Autodesk Fusion 360 part; units mm, degrees
sketch "Sketch1" plane through (0, 0, 0) normal (0, 0, 1) x (1, 0, 0)
  line L0 (4, -7) -> (-4, -7)
  line L1 (-4, -7) -> (-4, 7)
  line L2 (-4, 7) -> (4, 7)
  line L3 (4, 7) -> (4, -7)
  line L4 (4, -7) -> (-4, 7) construction
  line L5 (-4, -7) -> (4, 7) construction
  line L6 (0.5, -0.1) -> (-0.5, -0.1)
  line L7 (-0.5, -0.1) -> (-0.5, 0.1)
  line L8 (-0.5, 0.1) -> (0.5, 0.1)
  line L9 (0.5, 0.1) -> (0.5, -0.1)
  line L10 (0.5, -0.1) -> (-0.5, 0.1) construction
  line L11 (-0.5, -0.1) -> (0.5, 0.1) construction
  line L12 (0.5, -6.6) -> (-0.5, -6.6)
  line L13 (-0.5, -6.6) -> (-0.5, -6.4)
  line L14 (0.5, -6.4) -> (0.5, -6.6)
  line L15 (-0.5, -6.4) -> (0.5, -6.4)
  line L16 (2.959, -3.35) -> (1.959, -3.35)
  line L17 (1.959, -3.35) -> (1.959, -3.15)
  line L18 (2.959, -3.15) -> (2.959, -3.35)
  line L19 (1.959, -3.15) -> (2.959, -3.15)
  line L20 (2.959, 3.15) -> (1.959, 3.15)
  line L21 (1.959, 3.15) -> (1.959, 3.35)
  line L22 (2.959, 3.35) -> (2.959, 3.15)
  line L23 (1.959, 3.35) -> (2.959, 3.35)
  line L24 (0.5, 6.4) -> (-0.5, 6.4)
  line L25 (-0.5, 6.4) -> (-0.5, 6.6)
  line L26 (0.5, 6.6) -> (0.5, 6.4)
  line L27 (-0.5, 6.6) -> (0.5, 6.6)
  dimension "d61" = 8
  dimension "d62" = 14
  dimension "d63" = 1
  dimension "d64" = 0.2
  dimension "d67" = 2.459
  dimension "d68" = 6.5
extrude "Extrude1" add sketch "Sketch1" along normal blind 16 contours L6 L7 L8 L9 | L12 L13 L14 L15 | L16 L17 L18 L19 | L20 L21 L22 L23 | L24 L25 L26 L27 makes body 1 at (0.1667, -0.1, 5.3333) makes body 2 at (2.6257, 3.15, 5.3333) makes body 3 at (2.6257, -3.35, 5.3333) makes body 4 at (0.1667, 6.4, 5.3333) makes body 5 at (0.1667, -6.6, 5.3333)
extrude "Extrude2" add sketch "Sketch1" along normal blind 12.2 bodies 1 2 3 4 5
sketch "Sketch2" plane through (0, -7, 0) normal (0, -1, 0) x (1, 0, 0)
  line L0 (-4, 0) -> (4, 0)
  line L1 (4, 0) -> (4, 12.2)
  line L2 (4, 12.2) -> (-4, 12.2)
  line L3 (-4, 12.2) -> (-4, 0)
  circle A0 centre (0.7, 6) radius 3
  circle A1 centre (0.7, 6) radius 2
  line L4 (4, 0) -> (-4, 0)
  dimension "d73" = 6
  dimension "d74" = -1
  dimension "d76" = 3.3
  dimension "d78" = 6
extrude "Extrude3" add sketch "Sketch2" along normal blind 4 contours A0 bodies 1
extrude "Extrude4" cut sketch "Sketch2" against normal blind 12 contours A1 bodies 1
Part model, mm, in its own coordinate system. A direction names the side the tool comes from. Round coordinates to 2 decimals unless told otherwise and drop trailing zeros. Write each loop counter-clockwise with the first axis right and the second up, starting at its lowest first coordinate (ties: lowest second). Pieces come first, ordered by that corner, then holes. Notation, with made-up numbers: (72.25, 10) -> (123.25, 10) arc R21 ccw to (123.25, 25) -> close; hole circle Ø1 at (74, 18.25). An arc over 180 degrees is marked (long way). Return JSON: item names as keys, results as strings. Group by question number.
Q1. Pin check, flat tips, straight feed: pin 1 (0.8 mm diameter, centred on x = 0, z = 14.5, fed in from -Y); pin 2 (3 mm diameter, centred on x = 0.7, z = 6, fed in from -Y); pin 3 (0.8 mm diameter, centred on x = 2.5, z = 13, fed in from -Y). Stop position of each tip, or through.
Q2. Saw through at D-D on z = 6. Write the cut outline in (x, y), plus the area to 3 significant figures.
Q3. Mould opens along Y. For faces 1 (the flat face through (2.5, -3.15, 14.1)), 2 (the cylindrical face through (-0.9, -2.9, 7.2)), 3 (the flat face through (0, 7, 6)), 4 (the flat face through (-1, 0, 12.2)) say: pulls with the +Y half, pulls with the -Y half, needs draft (parallel to the pull), parting line crosses it, or undercut.
Q4. Saw through at A-A on z = 13.75. Write the cut outline in (x, y), plus the area to 4 significant figures.
Q5. Which spindle directions (+Z, -Z, +X, -X, +Y, -Y) get a long thin tool onto all of the face, cutting with end or side? Do faces 5 (the flat face through (0, 6.4, 14)), 6 (the flat face through (2.5, 3.35, 14.1)), 7 (the flat face through (0, -6.6, 14)). Say none if no direction does.
Q6. Saw through at C-C on x = -2. Write the cut outline in (y, z).
Q7. Probe L1, parallel to Z at x = 0.7, y = -6; L2, parallel to Y at x = 2.25, z = 3; L3, parallel to Z at x = 2.75, y = -3. List the from-to ranges inside material, lowest first. Write a range as [from, to].
Q8. Saw through at B-B on y = -4.5. Write the cut outline in (x, z), plus the area to 3 significant figures.
Answer:
{
 "1": {"pin 1": "y = -6.6", "pin 2": "y = 5", "pin 3": "y = -3.35"},
 "2": {"outline": "(-4, -7) -> (-2.3, -7) -> (-2.3, -11) -> (-1.3, -11) -> (-1.3, 5) -> (2.7, 5) -> (2.7, -11) -> (3.7, -11) -> (3.7, -7) -> (4, -7) -> (4, 7) -> (-4, 7) -> close", "area": "72.0 mm2"},
 "3": {"face 1": "undercut", "face 2": "needs draft", "face 3": "pulls with the +Y half", "face 4": "undercut"},
 "4": {"outline": "(-0.5, -6.6) -> (0.5, -6.6) -> (0.5, -6.4) -> (-0.5, -6.4) -> close; (-0.5, -0.1) -> (0.5, -0.1) -> (0.5, 0.1) -> (-0.5, 0.1) -> close; (-0.5, 6.4) -> (0.5, 6.4) -> (0.5, 6.6) -> (-0.5, 6.6) -> close; (1.96, -3.35) -> (2.96, -3.35) -> (2.96, -3.15) -> (1.96, -3.15) -> close; (1.96, 3.15) -> (2.96, 3.15) -> (2.96, 3.35) -> (1.96, 3.35) -> close", "area": "1.000 mm2"},
 "5": {"face 5": "+Z, +X, -X", "face 6": "+Z, +X, -X, +Y", "face 7": "+Z, +X, -X, -Y"},
 "6": {"outline": "(-11, 4.69) -> (-7, 4.69) -> (-7, 0) -> (7, 0) -> (7, 12.2) -> (-7, 12.2) -> (-7, 7.31) -> (-11, 7.31) -> close"},
 "7": {"L1": "[0, 4], [8, 12.2]", "L2": "[-7, 7]", "L3": "[0, 12.2]"},
 "8": {"outline": "(-4, 0) -> (4, 0) -> (4, 12.2) -> (-4, 12.2) -> close; hole circle Ø4 at (0.7, 6)", "area": "85.0 mm2"}
}
